```python
from build123d import *

# Parameters (mm, degrees)
F1_DEPTH = 1.6
F2_R     = 1.5
F3_DEPTH = 1.6
F4_R     = 1.5
F5_DEPTH = 1.6
F6_R     = 4.5
F6_R_2   = 1.5
F7_DEPTH = 1.6


with BuildPart() as f1:
    # F0 (on Top) → F1 (new body)
    with BuildSketch(Plane.XY):
        with BuildLine():
            Line((-39, -27), (39, -27))
            ThreePointArc((39, -27), (41.12132, -26.12132), (42, -24))
            Line((42, -24), (42, 24))
            ThreePointArc((42, 24), (41.12132, 26.12132), (39, 27))
            Line((39, 27), (-39, 27))
            ThreePointArc((-39, 27), (-41.12132, 26.12132), (-42, 24))
            Line((-42, 24), (-42, -24))
            ThreePointArc((-42, -24), (-41.12132, -26.12132), (-39, -27))
        make_face()
    extrude(amount=F1_DEPTH)

    # F2 (on face) → F3 (cut, through all)
    with BuildSketch(Plane.XY.offset(1.6)):
        with BuildLine():
            ThreePointArc((-40.56066, 25.56066), (-40.074025, 23.114181), (-38, 24.5))
            ThreePointArc((-38, 24.5), (-38.925975, 25.885819), (-40.56066, 25.56066))
        make_face()
        with Locations((18.5, 24.5)):
            Circle(F2_R)
        with Locations((18.5, -24.5)):
            Circle(F2_R)
        with Locations((-39.5, -24.5)):
            Circle(F2_R)
    extrude(amount=-F3_DEPTH, mode=Mode.SUBTRACT)

    # F4 (on face) → F5 (cut, through all)
    with BuildSketch(Plane.XY.offset(1.6)):
        with Locations((33.5, 24)):
            Circle(F4_R)
        with Locations((33.5, -24)):
            Circle(F4_R)
        with Locations((-32.5, 21)):
            Circle(F4_R)
        with Locations((-32.5, -21)):
            Circle(F4_R)
    extrude(amount=-F5_DEPTH, mode=Mode.SUBTRACT)

    # F6 (on face) → F7 (join)
    with BuildSketch(Plane.XY.offset(1.6)):
        with Locations((-39.5, 24.5)):
            Circle(F6_R)
        with Locations((-39.5, 24.5)):
            Circle(F6_R_2, mode=Mode.SUBTRACT)
        with Locations((-39.5, -24.5)):
            Circle(F6_R)
        with Locations((-39.5, -24.5)):
            Circle(F6_R_2, mode=Mode.SUBTRACT)
        with Locations((18.5, 24.5)):
            Circle(F6_R)
        with Locations((18.5, 24.5)):
            Circle(F6_R_2, mode=Mode.SUBTRACT)
        with Locations((18.5, -24.5)):
            Circle(F6_R)
        with Locations((18.5, -24.5)):
            Circle(F6_R_2, mode=Mode.SUBTRACT)
        with Locations((33.5, -24)):
            Circle(F6_R)
        with Locations((33.5, -24)):
            Circle(F6_R_2, mode=Mode.SUBTRACT)
        with Locations((33.5, 24)):
            Circle(F6_R)
        with Locations((33.5, 24)):
            Circle(F6_R_2, mode=Mode.SUBTRACT)
    extrude(amount=-F7_DEPTH)


solid = f1.part
```
The model under review builds one solid part; all positions refer to its coordinate system, in mm. A direction names the side the tool comes from. Give positions to 0.01 mm unless a question says otherwise; leave off trailing zeros. Order: outer loops, then holes, each group sorted by start corner. A loop starts at its lowest first (then second) coordinate and runs counter-clockwise, first axis right, second up. Notation, with made-up numbers: (84, 57.5) - (93, 57.5) arc R34 ccw to (93, 93.5) - close; hole circle Ø2 at (-17.75, 12.25). An arc over 180 degrees is marked (long way). Use CSV: the item, a comma, the result in double quotes. Start each with the question number.
Q1. We need section A-A, the plane x = -32.5. Write out the cut boundary in (y, z).
Q2. The part is to be moulded in two halves that separate along Y. For faces 1 (the cylindrical face through (18.4, -29, 0.8)), 2 (the flat face through (42, 0, 1)), 3 (the cylindrical face through (-33.61, 22.01, 0.81)), 4 (the flat face through (38, 27, 1)), say which applies: +Y half, -Y half, draft (parallel to the pull), parting line (faces both ways), or undercut.
Q3. We need section D-D, the plane y = 17. Write out the cut boundary in (x, z), and give its area (3 significant figures).
Q4. To check wall thickness, follow line 1 along Y through (x, z) = (18.5, 1.2); line 2 along Y through (x, z) = (-32.5, 1.25); line 3 along X through (y, z) = (12, 1.3). State the ranges of each line that lie inside material, in increasing order. Write a range as [from, to].
Q5. Clearance check with flat-ended pins moving along their axes: pin 1 Ø3.5 at (x, y) = (-39.5, -24.5) entering from -Z; pin 2 Ø2.5 at (x, y) = (-32.5, -21) entering from -Z; pin 3 Ø0.8 at (x, z) = (38, 0.5) entering from +Y; pin 4 Ø0.5 at (x, z) = (-13.5, 0.5) entering from -Y. State where each tip first meets the part, or that it passes through.
Q6. We need section C-C, the plane x = 18.5. Write out the cut boundary in (y, z).
Q7. We need section B-B, the plane z = 0.65. State how many separate pieces and enclosed holes the cut face has, and give its area (3 significant figures).
Q8. Tool access review of faces 5 (the flat face through (-11, -27, 1)), 6 (the flat face through (38, -27, 1)), 7 (the cylindrical face through (32.39, -22.99, 0.81)): name each direction out of +Z, -Z, +X, -X, +Y, -Y from which nothing blocks a thin tool from reaching the whole face with its end or side.
Outcome:
1,outline,"(-27, 0) - (-22.5, 0) - (-22.5, 1.6) - (-27, 1.6) - close; (-19.5, 0) - (19.5, 0) - (19.5, 1.6) - (-19.5, 1.6) - close; (22.5, 0) - (27, 0) - (27, 1.6) - (22.5, 1.6) - close"
2,face 1,"-Y half"
2,face 2,"draft"
2,face 3,"undercut"
2,face 4,"+Y half"
3,outline,"(-42, 0) - (42, 0) - (42, 1.6) - (-42, 1.6) - close"
3,area,"134 mm^2"
4,line 1,"y = [-29, -26], [-23, 23], [26, 29]"
4,line 2,"y = [-27, -22.5], [-19.5, 19.5], [22.5, 27]"
4,line 3,"x = [-42, 42]"
5,pin 1,"stops at z = 0"
5,pin 2,"passes through"
5,pin 3,"stops at y = 27"
5,pin 4,"stops at y = -27"
6,outline,"(-29, 0) - (-26, 0) - (-26, 1.6) - (-29, 1.6) - close; (-23, 0) - (23, 0) - (23, 1.6) - (-23, 1.6) - close; (26, 0) - (29, 0) - (29, 1.6) - (26, 1.6) - close"
7,separate pieces,"1"
7,enclosed holes,"8"
7,area,"4,550 mm^2"
8,face 5,"+Z, -Z, -Y"
8,face 6,"+Z, -Z, +X, -Y"
8,face 7,"+Z, -Z"
